Autodesk Inventor part; units mm, degrees
ref_plane "YZ Plane" through (0, 0, 0) normal (1, 0, 0) x (0, 1, 0)
ref_plane "XZ Plane" through (0, 0, 0) normal (0, 1, 0) x (-1, 0, 0)
ref_plane "XY Plane" through (0, 0, 0) normal (0, 0, 1) x (1, 0, 0)
sketch "Sketch1" plane through (0, 0, 0) normal (0, 0, 1) x (1, 0, 0)
  line L0 (-20.65, -25.5) -> (20.65, -25.5)
  line L1 (20.65, -25.5) -> (20.65, 25.5)
  line L2 (20.65, 25.5) -> (-20.65, 25.5)
  line L3 (-20.65, 25.5) -> (-20.65, -25.5)
  line L4 (-20.65, -25.5) -> (20.65, 25.5) construction
  line L5 (20.65, -25.5) -> (-20.65, 25.5) construction
  line L6 (0, 2.9) -> (0, 4.9) construction
  line L7 (16, 2.9) -> (16, 4.9)
  line L8 (-16, 4.9) -> (-16, 2.9)
  arc A0 (-16, 2.9) -> (16, 2.9) centre (0, 2.9) ccw
  arc A1 (16, 4.9) -> (-16, 4.9) centre (0, 4.9) ccw
  line L9 (-15.5, 20.4) -> (-15.5, 18.4) construction
  line L10 (-17.1, 20.4) -> (-17.1, 18.4)
  line L11 (-13.9, 18.4) -> (-13.9, 20.4)
  arc A2 (-13.9, 20.4) -> (-17.1, 20.4) centre (-15.5, 20.4) ccw
  arc A3 (-17.1, 18.4) -> (-13.9, 18.4) centre (-15.5, 18.4) ccw
  line L12 (15.5, 20.4) -> (15.5, 18.4) construction
  line L13 (13.9, 20.4) -> (13.9, 18.4)
  line L14 (17.1, 18.4) -> (17.1, 20.4)
  arc A4 (17.1, 20.4) -> (13.9, 20.4) centre (15.5, 20.4) ccw
  arc A5 (13.9, 18.4) -> (17.1, 18.4) centre (15.5, 18.4) ccw
  line L15 (15.5, -10.6) -> (15.5, -12.6) construction
  line L16 (13.9, -10.6) -> (13.9, -12.6)
  line L17 (17.1, -12.6) -> (17.1, -10.6)
  arc A6 (17.1, -10.6) -> (13.9, -10.6) centre (15.5, -10.6) ccw
  arc A7 (13.9, -12.6) -> (17.1, -12.6) centre (15.5, -12.6) ccw
  line L18 (-15.5, -10.6) -> (-15.5, -12.6) construction
  line L19 (-17.1, -10.6) -> (-17.1, -12.6)
  line L20 (-13.9, -12.6) -> (-13.9, -10.6)
  arc A8 (-13.9, -10.6) -> (-17.1, -10.6) centre (-15.5, -10.6) ccw
  arc A9 (-17.1, -12.6) -> (-13.9, -12.6) centre (-15.5, -12.6) ccw
  point P0 (0, 0)
  point P1 (0, 3.9)
  point P2 (-15.5, 19.4)
  point P3 (15.5, 19.4)
  point P4 (15.5, -11.6)
  point P5 (-15.5, -11.6)
  dimension "d0" = 51
  dimension "d1" = 41.3
  dimension "d2" = 28.4
  dimension "d3" = 2
  dimension "d4" = 16
  dimension "d5" = 2
  dimension "d6" = 31
  dimension "d7" = 31
  dimension "d8" = 1.6
  dimension "d10" = 15.5
  dimension "d11" = 15.5
  dimension "d22" = 51
extrude "Extrusion1" add sketch "Sketch1" along normal blind 3
sketch "Sketch2" plane through (-20.65, -25.5, 0) normal (0, -1, 0) x (1, 0, 0)
  line L0 (41.3, 0) -> (41.3, 3)
  line L1 (0, 0) -> (41.3, 0)
  line L2 (41.3, 0) -> (41.3, 53)
  line L3 (41.3, 53) -> (0, 53)
  line L4 (0, 53) -> (0, 0)
  line L5 (5.65, 11.5) -> (5.65, 41.5) construction
  line L6 (3.5, 11.5) -> (3.5, 41.5)
  line L7 (7.8, 41.5) -> (7.8, 11.5)
  arc A0 (3.5, 11.5) -> (7.8, 11.5) centre (5.65, 11.5) ccw
  arc A1 (7.8, 41.5) -> (3.5, 41.5) centre (5.65, 41.5) ccw
  line L8 (35.65, 11.5) -> (35.65, 41.5) construction
  line L9 (33.5, 11.5) -> (33.5, 41.5)
  line L10 (37.8, 41.5) -> (37.8, 11.5)
  arc A2 (33.5, 11.5) -> (37.8, 11.5) centre (35.65, 11.5) ccw
  arc A3 (37.8, 41.5) -> (33.5, 41.5) centre (35.65, 41.5) ccw
  line L11 (0, 26.5) -> (5.65, 26.5) construction
  line L12 (5.65, 26.5) -> (35.65, 26.5) construction
  line L13 (20.65, 26.5) -> (20.65, 53) construction
  point P0 (20.65, 0)
  dimension "d14" = 53
  dimension "d23" = 4.3
  dimension "d24" = 30
  dimension "d25" = 30
extrude "Extrusion3" add sketch "Sketch2" against normal blind 3
chamfer "Chamfer1" distance 3 angle 45 4 edges at (20.65, 25.5, 1.5) (-20.65, 25.5, 1.5) (-20.65, -24, 53) (20.65, -24, 53)
properties part number "StepperMount"
Design review of the part built by this model. Coordinates are the model's own, in mm. A direction names the side the tool comes from. Coordinates: 2 decimals unless noted, no trailing zeros. Loops run counter-clockwise (first coordinate to the right, second up) from the corner with the lowest first, then second, coordinate; pieces in that order, holes last. Notation, with made-up numbers: (-36.75, 79.5) -> (-11.75, 79.5) arc R11 ccw to (-11.75, 96.5) -> close; hole circle Ø1 at (-24, -20). An arc over 180 degrees is marked (long way). Use a Markdown table: item, result. Add a question column.
Item 1: We need section D-D, the plane y = -11.5. Write out the cut boundary in (x, z).
Item 2: We need section A-A, the plane z = 25.5. Write out the cut boundary in (x, y), and give its area (3 significant figures).
Item 3: Machinability: for faces 1 (the flat face through (12.85, -24, 26)), 2 (the cylindrical face through (15.5, 22, 1.5)), 3 (the flat face through (-20.65, -23, 14)), which of the approach directions +Z, -Z, +X, -X, +Y, -Y give a long, thin tool a straight path to every point of the face, cutting with its end or side? Answer none if there is none.
Item 4: Clearance check with flat-ended pins moving along their axes: P1, Ø10, axis at x = -16, z = 36.5, coming from the +Y side; P2, Ø12, axis at x = -4.5, y = 7, coming from the -Z side; P3, Ø12, axis at x = -11, y = 12.5, coming from the +Z side. State where each tip first meets the part, or that it passes through.
Item 5: Wall thickness on L1, parallel to Y at x = -6, z = 42; L2, parallel to Z at x = 10, y = -19: over which ranges is each line inside the solid? List them lowest first. Write a range as from..to.
Item 6: We need section B-B, the plane x = 0. Write out the cut boundary in (y, z), and give its area (3 significant figures).
Item 7: We need section C-C, the plane y = 14.5. Write out the cut boundary in (x, z).
Item 8: The part is to be moulded in two halves that separate along Y. For faces 4 (the flat face through (-9, -11, 0)), 5 (the flat face through (16, 4, 1)), say which applies: +Y half, -Y half, draft (parallel to the pull), parting line (faces both ways), or undercut.
Numbers:
| question | item | result |
|---|---|---|
| 1 | outline | (-20.65, 0) -> (-17.1, 0) -> (-17.1, 3) -> (-20.65, 3) -> close; (-13.9, 0) -> (-6.97, 0) -> (-6.97, 3) -> (-13.9, 3) -> close; (6.97, 0) -> (13.9, 0) -> (13.9, 3) -> (6.97, 3) -> close; (17.1, 0) -> (20.65, 0) -> (20.65, 3) -> (17.1, 3) -> close |
| 2 | outline | (-20.65, -25.5) -> (-17.15, -25.5) -> (-17.15, -22.5) -> (-20.65, -22.5) -> close; (-12.85, -25.5) -> (12.85, -25.5) -> (12.85, -22.5) -> (-12.85, -22.5) -> close; (17.15, -25.5) -> (20.65, -25.5) -> (20.65, -22.5) -> (17.15, -22.5) -> close |
| 2 | area | 98.1 mm^2 |
| 3 | face 1 | +Y, -Y |
| 3 | face 2 | +Z, -Z |
| 3 | face 3 | +Z, -Z, -X, +Y, -Y |
| 4 | P1 | stops at y = -22.5 |
| 4 | P2 | passes through |
| 4 | P3 | stops at z = 3 |
| 5 | L1 | y = -25.5..-22.5 |
| 5 | L2 | z = 0..3 |
| 6 | outline | (-25.5, 0) -> (-13.1, 0) -> (-13.1, 3) -> (-22.5, 3) -> (-22.5, 53) -> (-25.5, 53) -> close; (20.9, 0) -> (25.5, 0) -> (25.5, 3) -> (20.9, 3) -> close |
| 6 | area | 201 mm^2 |
| 7 | outline | (-20.65, 0) -> (-12.8, 0) -> (-12.8, 3) -> (-20.65, 3) -> close; (12.8, 0) -> (20.65, 0) -> (20.65, 3) -> (12.8, 3) -> close |
| 8 | face 4 | draft |
| 8 | face 5 | undercut |
